from build123d import *

# Parameters (mm, degrees)
SKETCH1_W                   = 100
SKETCH1_H                   = 68
BOSS_EXTRUDE1_DEPTH         = 40
FILLET1_R                   = 10
CUT_EXTRUDE1_REACH          = 74.498
M6_TAPPED_HOLE1_D           = 5
M6_TAPPED_HOLE1_DEPTH       = 17
M6_TAPPED_HOLE1_CSINK_D     = 6.05
M6_TAPPED_HOLE1_CSINK_ANGLE = 90
M6_TAPPED_HOLE1_TIP         = 1.502151548


with BuildPart() as part:
    # Sketch1 → Boss-Extrude1 (new body)
    with BuildSketch(Plane(origin=(0, 0, 0), x_dir=(1, 0, 0), z_dir=(0, 1, 0))):
        Rectangle(SKETCH1_W, SKETCH1_H)
    extrude(amount=-BOSS_EXTRUDE1_DEPTH)

    # Fillet1
    fillet1_edges = [part.edges().sort_by_distance(p)[0] for p in [
        (50, -20, 34),
        (-50, -20, 34),
        (-50, -20, -34),
        (50, -20, -34),
    ]]
    fillet(fillet1_edges, radius=FILLET1_R)

    # Sketch2 → Cut-Extrude1 (cut, up to next)
    with BuildSketch(Plane(origin=(0, 0, 0), x_dir=(1, 0, 0), z_dir=(0, 1, 0)), mode=Mode.PRIVATE) as cut_extrude1_sk1:
        with BuildLine():
            Line((-32.625, -21.36), (32.625, -21.36))
            ThreePointArc((32.625, -21.36), (34.908954903, -20.413954903), (35.855, -18.13))
            Line((35.855, -18.13), (35.855, 18.13))
            ThreePointArc((35.855, 18.13), (34.908954903, 20.413954903), (32.625, 21.36))
            Line((32.625, 21.36), (24.265, 21.36))
            Line((24.265, 21.36), (24.265, 15))
            ThreePointArc((24.265, 15), (22.575006127, 10.919993873), (18.495, 9.23))
            Line((18.495, 9.23), (14.495, 9.23))
            ThreePointArc((14.495, 9.23), (12.211045097, 8.283954903), (11.265, 6))
            Line((11.265, 6), (11.265, -10.13))
            ThreePointArc((11.265, -10.13), (5.495, -15.9), (-0.275, -10.13))
            Line((-0.275, -10.13), (-0.275, 6))
            ThreePointArc((-0.275, 6), (-1.221045097, 8.283954903), (-3.505, 9.23))
            Line((-3.505, 9.23), (-7.505, 9.23))
            ThreePointArc((-7.505, 9.23), (-11.585006127, 10.919993873), (-13.275, 15))
            Line((-13.275, 15), (-13.275, 21.36))
            Line((-13.275, 21.36), (-32.625, 21.36))
            ThreePointArc((-32.625, 21.36), (-34.908954903, 20.413954903), (-35.855, 18.13))
            Line((-35.855, 18.13), (-35.855, -18.13))
            ThreePointArc((-35.855, -18.13), (-34.908954903, -20.413954903), (-32.625, -21.36))
        make_face()
    cut_extrude1_tool1 = extrude(cut_extrude1_sk1.sketch, amount=-CUT_EXTRUDE1_REACH, mode=Mode.PRIVATE) & part.part
    add(cut_extrude1_tool1.solids().sort_by_distance((-1.698637, 0, 2.611892))[0], mode=Mode.SUBTRACT)

    # Cut-Sweep1: sweep along a path in Sketch5
    with BuildLine(Plane(origin=(0, 0, 0), x_dir=(1, 0, 0), z_dir=(0, 1, 0))) as cut_sweep1_path:
        Line((-32.625, -21.36), (32.625, -21.36))
        ThreePointArc((32.625, -21.36), (34.908954903, -20.413954903), (35.855, -18.13))
        Line((35.855, -18.13), (35.855, 18.13))
        ThreePointArc((35.855, 18.13), (34.908954903, 20.413954903), (32.625, 21.36))
        Line((32.625, 21.36), (24.265, 21.36))
        Line((24.265, 21.36), (24.265, 15))
        ThreePointArc((24.265, 15), (22.575006127, 10.919993873), (18.495, 9.23))
        Line((18.495, 9.23), (14.495, 9.23))
        ThreePointArc((14.495, 9.23), (12.211045097, 8.283954903), (11.265, 6))
        Line((11.265, 6), (11.265, -10.13))
        ThreePointArc((11.265, -10.13), (5.495, -15.9), (-0.275, -10.13))
        Line((-0.275, -10.13), (-0.275, 6))
        ThreePointArc((-0.275, 6), (-1.221045097, 8.283954903), (-3.505, 9.23))
        Line((-3.505, 9.23), (-7.505, 9.23))
        ThreePointArc((-7.505, 9.23), (-11.585006127, 10.919993873), (-13.275, 15))
        Line((-13.275, 15), (-13.275, 21.36))
        Line((-13.275, 21.36), (-32.625, 21.36))
        ThreePointArc((-32.625, 21.36), (-34.908954903, 20.413954903), (-35.855, 18.13))
        Line((-35.855, 18.13), (-35.855, -18.13))
        ThreePointArc((-35.855, -18.13), (-34.908954903, -20.413954903), (-32.625, -21.36))
    # Sketch3 → Cut-Sweep1 (sweep, cut)
    with BuildSketch(Plane.XY):
        Polygon((35.855, -3.2), (36.818641914, -40), (34.855, -40), (34.855, -3.2), align=None)
    sweep(path=cut_sweep1_path.line, transition=Transition.RIGHT, mode=Mode.SUBTRACT)

    # M6 Tapped Hole1
    with Locations(Plane(origin=(0, -40, 0), x_dir=(-1, 0, 0), z_dir=(0, -1, 0))):
        with Locations((-43, 27), (43, 27), (43, -27), (-43, -27)):
            CounterSinkHole(M6_TAPPED_HOLE1_D / 2, M6_TAPPED_HOLE1_CSINK_D / 2, depth=M6_TAPPED_HOLE1_DEPTH, counter_sink_angle=M6_TAPPED_HOLE1_CSINK_ANGLE)
            with Locations((0, 0, -(M6_TAPPED_HOLE1_DEPTH + M6_TAPPED_HOLE1_TIP / 2))):  # 118° drill point
                Cone(0, M6_TAPPED_HOLE1_D / 2, M6_TAPPED_HOLE1_TIP, mode=Mode.SUBTRACT)


solid = part.part
Design review of the part built by this model. Coordinates are the model's own, in mm. A direction names the side the tool comes from. Round coordinates to 2 decimals unless told otherwise and drop trailing zeros. Order: outer loops, then holes, each group sorted by start corner. A loop starts at its lowest first (then second) coordinate and runs counter-clockwise, first axis right, second up. Notation, with made-up numbers: M 9,34 L 63,34 A16 cw 63,49 Z; hole C -1,-11.75 d11. An arc over 180 degrees is marked long. Answer as CSV lines item,"result". Start each with the question number.
1) For pin 1 Ø3 at (x, z) = (43, -27) entering from -Y, flat-tipped, find the tip position at first contact; note if it passes through.
2) Add section C-C (y = -33). Give the number of separate pieces and of enclosed holes in the cut face, then the cut area to 3 significant figures.
3) Add section A-A (x = 17). Give the boundary of the cut face in (y, z).
4) The part is to be moulded in two halves that separate along X. For faces 1 (the face through (47.15, -20.28, -30.99)), 2 (the face through (0, -2, 21.36)), say which applies: +X half, -X half, draft (parallel to the pull), parting line (faces both ways), or undercut.
5) Wall thickness on line 1 along X through (y, z) = (-10, 2.5); line 2 along Z through (x, y) = (-43, -28); line 3 along X through (y, z) = (-30, -27): over which ranges is each line inside the solid? List them lowest first. Write a range as [from, to].
6) Add section D-D (y = -14). Give the boundary of the cut face in (x, z) (3 decimals).
7) Add section B-B (z = 0). Give the boundary of the cut face in (x, y) (3 decimals).
8) Tool access review of faces 3 (the face through (17, -2, -9.23)), 4 (the face through (-40.615, -31.122, -27.751)), 5 (the face through (46.99, -20.28, 31.15)): name each direction out of +Z, -Z, +X, -X, +Y, -Y from which nothing blocks a thin tool from reaching the whole face with its end or side.
Resolved:
1,pin 1,"y = -22.4"
2,separate pieces,"1"
2,enclosed holes,"5"
2,area,"4,080 mm^2"
3,outline,"M -40,-34 L 0,-34 L 0,-9.23 L -3.2,-9.23 L -40,-10.19 Z; M -40,22.32 L -3.2,21.36 L 0,21.36 L 0,34 L -40,34 Z"
4,face 1,"+X half"
4,face 2,"undercut"
5,line 1,"[-50, -36.03], [-0.1, 11.09], [36.03, 50]"
5,line 2,"[-33.54, -29.5], [-24.5, 24.5], [29.5, 33.54]"
5,line 3,"[-49.54, -45.5], [-40.5, 40.5], [45.5, 49.54]"
6,outline,"M -50,-24 A10 ccw -40,-34 L 40,-34 A10 ccw 50,-24 L 50,24 A10 ccw 40,34 L -40,34 A10 ccw -50,24 Z; hole M -36.138,-18.13 A3.513 ccw -32.625,-21.643 L -12.992,-21.643 L -12.992,-15 A5.487 cw -7.505,-9.513 L -3.505,-9.513 A3.513 ccw 0.008,-6 L 0.008,10.13 A5.487 cw 10.982,10.13 L 10.982,-6 A3.513 ccw 14.495,-9.513 L 18.495,-9.513 A5.487 cw 23.982,-15 L 23.982,-21.643 L 32.625,-21.643 A3.513 ccw 36.138,-18.13 L 36.138,18.13 A3.513 ccw 32.625,21.643 L -32.625,21.643 A3.513 ccw -36.138,18.13 Z"
7,outline,"M -50,-40 L -36.819,-40 L -35.855,-3.2 L -35.855,0 L -50,0 Z; M -0.275,-3.2 L 0.689,-40 L 10.301,-40 L 11.265,-3.2 L 11.265,0 L -0.275,0 Z; M 35.855,-3.2 L 36.819,-40 L 50,-40 L 50,0 L 35.855,0 Z"
8,face 3,"+Y, -Y"
8,face 4,"-Y"
8,face 5,"+Z, +X, +Y, -Y"
